Could you check a few things on this model? Use its own coordinates, in mm. Give positions to 0.01 mm unless a question says otherwise; leave off trailing zeros. Loops run counter-clockwise (first coordinate to the right, second up) from the corner with the lowest first, then second, coordinate; pieces in that order, holes last. Notation, with made-up numbers: M 83.5,-15 L 133.5,-15 A24 cw 133.5,21 Z; hole C 89,-12.75 d3. An arc over 180 degrees is marked long. Answer in a Markdown table with one row per item. Add a question column.
1. I'm going to push flat-ended pins straight in: pin 1 Ø1 at (x, y) = (-10, 43.5) entering from -Z; pin 2 Ø1.5 at (x, z) = (-21.5, 1) entering from -Y; pin 3 Ø1.5 at (x, y) = (-10, 111.5) entering from -Z. Where does each tip first touch, or does it pass through?
2. If we section it at D-D on z = 2.2: List the corners of the cut face in (x, y) for me.
3. If we section it at B-B on y = 138.5: List the corners of the cut face in (x, z) for me, then the cut area to 3 significant figures.
4. If we section it at A-A on x = -10: List the corners of the cut face in (y, z) for me, then the cut area to 3 significant figures.
5. I need wall thicknesses on line 1 along X through (y, z) = (138.5, 1.45); line 2 along X through (y, z) = (70.5, 2.2); line 3 along X through (y, z) = (46, 0.8). Which ranges of each line are inside material? Lowest first, please. Write a range as from..to.
6. If we section it at C-C on y = 32: List the corners of the cut face in (x, z) for me.
Autodesk Inventor part; units mm, degrees
ref_plane "YZ Plane" through (0, 0, 0) normal (1, 0, 0) x (0, 1, 0)
ref_plane "XZ Plane" through (0, 0, 0) normal (0, 1, 0) x (-1, 0, 0)
ref_plane "XY Plane" through (0, 0, 0) normal (0, 0, 1) x (1, 0, 0)
sketch "Szkic1" plane through (0, 0, 0) normal (0, 0, 1) x (1, 0, 0)
  line L0 (-10, 0) -> (-10, 0)
  line L1 (-20, 10) -> (-20, 107)
  line L2 (0, 107) -> (0, 10)
  arc A0 (-20, 10) -> (-10, 0) centre (-10, 10) ccw
  arc A1 (-10, 0) -> (0, 10) centre (-10, 10) ccw
  line L3 (-23, 143) -> (-23, 107)
  line L4 (3, 107) -> (3, 143)
  line L5 (3, 143) -> (-23, 143)
  line L6 (-23, 143) -> (3, 107) construction
  line L7 (-23, 107) -> (3, 143) construction
  line L8 (-23, 107) -> (-20, 107)
  line L9 (0, 107) -> (3, 107)
  arc A2 (-7.6923, 124.4615) -> (-12.3077, 124.4615) centre (-10, 130) ccw
  arc A3 (-12.3077, 124.4615) -> (-7.6923, 124.4615) centre (-10, 123.5) ccw
  circle A4 centre (-10, 111.5) radius 1.25
  circle A5 centre (-10, 138.5) radius 1.25
  point P0 (0, 0)
  point P1 (-10, 125)
  dimension "d2" = 10
  dimension "d3" = 26
  dimension "d4" = 36
  dimension "d5" = 20
  dimension "d10" = 3
  dimension "d13" = 5
  dimension "d19" = 2.5
  dimension "d20" = 2.5
  dimension "d22" = 6
  dimension "d23" = 13
  dimension "d24" = 13
  dimension "d25" = 6.5
  dimension "d26" = 13
  dimension "d27" = 4.5
  dimension "d28" = 31.5
  dimension "d29" = 13
  dimension "d30" = 120
  dimension "d31" = 36
extrude "Wyciągnięcie proste1" add sketch "Szkic1" along normal blind 3
sketch "Szkic2" plane through (0, 0, 3) normal (0, 0, 1) x (1, 0, 0)
  point P0 (0, 0)
  point P1 (-10, 32)
  point P2 (-10, 70.5805)
  dimension "d49" = 32
hole "Otwór1" at (-10, 32, 3) at (-10, 70.5805, 3) direction (0, 0, -1) diameter 3.2 end through all
sketch "Szkic3" plane through (0, 0, 3) normal (0, 0, 1) x (1, 0, 0)
  arc A0 (-20, 10) -> (0, 10) centre (-10, 10) ccw
  point P0 (0, 0)
  point P1 (-10, 102)
  dimension "d41" = 92
hole "Otwór2" at (-10, 102, 3) direction (0, 0, -1) diameter 3.2 end through all
sketch "Szkic4" plane through (0, 0, 3) normal (0, 0, 1) x (1, 0, 0)
  arc A0 (-20, 10) -> (0, 10) centre (-10, 10) ccw
  point P0 (0, 0)
properties material "Drewno (wiśnia)"
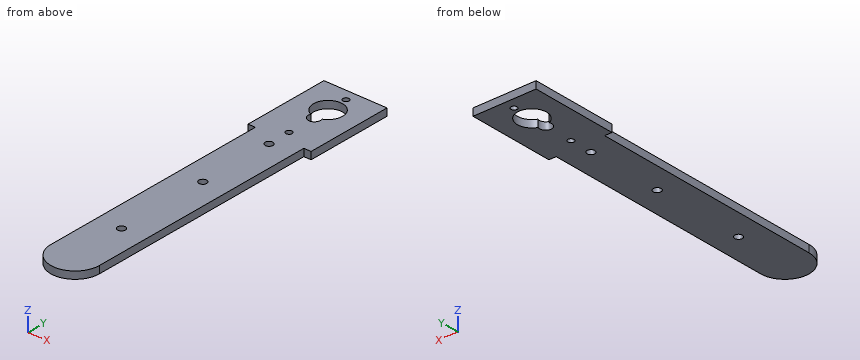
Results:
| question | item | result |
|---|---|---|
| 1 | pin 1 | z = 0 |
| 1 | pin 2 | y = 107 |
| 1 | pin 3 | through |
| 2 | outline | M -23,107 L -20,107 L -20,10 A10 ccw 0,10 L 0,107 L 3,107 L 3,143 L -23,143 Z; hole M -12.31,124.46 A2.5 ccw long -7.69,124.46 A6 ccw long Z; hole C -10,32 d3.2; hole C -10,70.58 d3.2; hole C -10,102 d3.2; hole C -10,111.5 d2.5; hole C -10,138.5 d2.5 |
| 3 | outline | M -23,0 L -11.25,0 L -11.25,3 L -23,3 Z; M -8.75,0 L 3,0 L 3,3 L -8.75,3 Z |
| 3 | area | 70.5 mm2 |
| 4 | outline | M 0,0 L 30.4,0 L 30.4,3 L 0,3 Z; M 33.6,0 L 68.98,0 L 68.98,3 L 33.6,3 Z; M 72.18,0 L 100.4,0 L 100.4,3 L 72.18,3 Z; M 103.6,0 L 110.25,0 L 110.25,3 L 103.6,3 Z; M 112.75,0 L 121,0 L 121,3 L 112.75,3 Z; M 136,0 L 137.25,0 L 137.25,3 L 136,3 Z; M 139.75,0 L 143,0 L 143,3 L 139.75,3 Z |
| 4 | area | 340 mm2 |
| 5 | line 1 | -23..-11.25, -8.75..3 |
| 5 | line 2 | -20..-11.6, -8.4..0 |
| 5 | line 3 | -20..0 |
| 6 | outline | M -20,0 L -11.6,0 L -11.6,3 L -20,3 Z; M -8.4,0 L 0,0 L 0,3 L -8.4,3 Z |
